Autodesk Inventor part; units mm, degrees
ref_plane "YZ Plane" through (0, 0, 0) normal (1, 0, 0) x (0, 1, 0)
ref_plane "XZ Plane" through (0, 0, 0) normal (0, 1, 0) x (-1, 0, 0)
ref_plane "XY Plane" through (0, 0, 0) normal (0, 0, 1) x (1, 0, 0)
sketch "Skizze1" plane through (0, 0, 0) normal (0, 1, 0) x (-1, 0, 0)
  line L0 (13.1, 3.4) -> (-13.1, 3.4)
  line L1 (-13.9, 2.6) -> (-13.9, -2.6)
  line L2 (-13.1, -3.4) -> (13.1, -3.4)
  line L3 (13.9, -2.6) -> (13.9, 2.6)
  line L4 (13.9, 3.4) -> (-13.9, -3.4) construction
  line L5 (-13.9, 3.4) -> (13.9, -3.4) construction
  arc A0 (13.9, 2.6) -> (13.1, 3.4) centre (13.1, 2.6) ccw
  arc A1 (13.1, -3.4) -> (13.9, -2.6) centre (13.1, -2.6) ccw
  arc A2 (-13.9, -2.6) -> (-13.1, -3.4) centre (-13.1, -2.6) ccw
  arc A3 (-13.1, 3.4) -> (-13.9, 2.6) centre (-13.1, 2.6) ccw
  line L6 (9.2, 0) -> (-9.2, 0) construction
  line L7 (9.2, -7.8) -> (-9.2, -7.8)
  line L8 (-9.2, 7.8) -> (9.2, 7.8)
  arc A4 (9.2, -7.8) -> (9.2, 7.8) centre (9.2, 0) ccw
  arc A5 (-9.2, 7.8) -> (-9.2, -7.8) centre (-9.2, 0) ccw
  point P0 (0, 0)
  dimension "d0" = 27.8
  dimension "d1" = 6.8
  dimension "d2" = 0.8
  dimension "d6" = 4.4
  dimension "d7" = 34
extrude "Extrusion1" add sketch "Skizze1" along normal mid plane 46.3
properties part number "Kupferspule" material "Kupfer"
Design review of the part built by this model. Coordinates are the model's own, in mm. A direction names the side the tool comes from. Coordinates: 2 decimals unless noted, no trailing zeros. Order: outer loops, then holes, each group sorted by start corner. A loop starts at its lowest first (then second) coordinate and runs counter-clockwise, first axis right, second up. Notation, with made-up numbers: (-26.75, 32) - (11.25, 32) arc R19 ccw to (11.25, 55) - close; hole circle Ø3 at (83.25, 21.25). An arc over 180 degrees is marked (long way). Put each result on its own line as item: value.
1) Take a section at C-C, the plane z = 0. Give the boundary of the cut face in (x, y), and give its area (3 significant figures).
Response values:
outline: (-17, -23.15) - (-13.9, -23.15) - (-13.9, 23.15) - (-17, 23.15) - close; (13.9, -23.15) - (17, -23.15) - (17, 23.15) - (13.9, 23.15) - close
area: 287 mm²
2) The part is to be moulded in two halves that separate along Z. For faces 1 (the face through (-13.9, 0, 0)), 2 (the face through (17, 0, 0)), 3 (the face through (0, 0, 7.8)), say which applies: released by +Z, released by -Z, zero draft, split by the parting line, or undercut.
Response values:
face 1: undercut
face 2: split by the parting line
face 3: released by +Z
3) Insertion check: P1, Ø5, axis at y = 12.5, z = 4, coming from the +X side; P2, Ø2, axis at y = -1, z = 5.5, coming from the +X side; P3, Ø3, axis at y = 3.5, z = -3.5, coming from the -X side. Each pin has a flat end and moves straight along its axis. Give the tip position at first contact, or say it passes through.
Response values:
P1: stops at x = 16.85
P2: stops at x = 15.57
P3: stops at x = -16.74
4) Take a section at D-D, the plane z = -5.75. Give the boundary of the cut face in (x, y), and give its area (3 significant figures).
Response values:
outline: (-14.47, -23.15) - (14.47, -23.15) - (14.47, 23.15) - (-14.47, 23.15) - close
area: 1,340 mm²
5) Take a section at A-A, the plane x = 3. Give the boundary of the cut face in (y, z), and give its area (3 significant figures).
Response values:
outline: (-23.15, -7.8) - (23.15, -7.8) - (23.15, -3.4) - (-23.15, -3.4) - close; (-23.15, 3.4) - (23.15, 3.4) - (23.15, 7.8) - (-23.15, 7.8) - close
area: 407 mm²
6) Take a section at B-B, the plane y = 4.5. Give the boundary of the cut face in (x, z), and give its area (3 significant figures).
Response values:
outline: (-9.2, -7.8) - (9.2, -7.8) arc R7.8 ccw to (9.2, 7.8) - (-9.2, 7.8) arc R7.8 ccw to start; hole (-13.9, -2.6) arc R0.8 ccw to (-13.1, -3.4) - (13.1, -3.4) arc R0.8 ccw to (13.9, -2.6) - (13.9, 2.6) arc R0.8 ccw to (13.1, 3.4) - (-13.1, 3.4) arc R0.8 ccw to (-13.9, 2.6) - close
area: 290 mm²
7) Wall thickness on L1, parallel to Z at x = 6, y = -15; L2, parallel to X at y = -12, z = 1.25; L3, parallel to X at y = -4, z = -2.5: over which ranges is each line inside the solid? List them lowest first. Write a range as from..to.
Response values:
L1: z = -7.8..-3.4, 3.4..7.8
L2: x = -16.9..-13.9, 13.9..16.9
L3: x = -16.59..-13.9, 13.9..16.59
8) Tool access review of faces 4 (the face through (13.9, 0, 0)), 5 (the face through (0, 0, -7.8)): name each direction out of +Z, -Z, +X, -X, +Y, -Y from which nothing blocks a thin tool from reaching the whole face with its end or side.
Response values:
face 4: +Y, -Y
face 5: -Z, +X, -X, +Y, -Y
